Autodesk Inventor part; units mm, degrees
ref_plane "YZ Plane" through (0, 0, 0) normal (1, 0, 0) x (0, 1, 0)
ref_plane "XZ Plane" through (0, 0, 0) normal (0, 1, 0) x (-1, 0, 0)
ref_plane "XY Plane" through (0, 0, 0) normal (0, 0, 1) x (1, 0, 0)
sketch "Esboço1" plane through (0, 0, 0) normal (0, 0, 1) x (1, 0, 0)
  circle A0 centre (0, 0) radius 25
  dimension "d0" = 50
extrude "Extrusão1" add sketch "Esboço1" along normal blind 20
fillet "Arredondamento1" radius 2 1 edges at (-25, 0, 20)
sketch "Esboço2" plane through (0, 0, 20) normal (0, 0, 1) x (1, 0, 0)
  circle A0 centre (0, 0) radius 2.5
  circle A1 centre (0, 18) radius 2.5
  dimension "d4" = 5
  dimension "d5" = 5
  dimension "d6" = 18
extrude "Extrusão2" cut sketch "Esboço2" against normal blind 15
chamfer "Chanfro1" distance 0.6 angle 45 2 edges at (-2.5, 0, 20) (-2.5, 18, 20)
pattern_circular "Padrão circular1" count 6 over 360 about axis through (0, 0, 0) along (0, 0, 1) of "Extrusão2", "Chanfro1"
sketch "Esboço3" plane through (0, 0, 0) normal (0, 0, -1) x (-1, 0, 0)
  arc A0 (3, 30) -> (-3, 30) centre (0, 30) ccw
  circle A1 centre (0, 30) radius 1.5
  line L0 (3, 30) -> (3, 24.3841)
  line L1 (-3, 30) -> (-3, 24.3841)
  line L2 (-3, 24.3841) -> (3, 24.3841)
  point P0 (0, 0)
  dimension "d15" = 6
  dimension "d16" = 3
  dimension "d17" = 30
extrude "Extrusão3" add sketch "Esboço3" against normal blind 5
mirror "Espelhamento1" about plane through (0, 0, 0) normal (0, 1, 0) of "Extrusão3"
sketch "Esboço4" plane through (0, 0, 20) normal (0, 0, 1) x (1, 0, 0)
  circle A0 centre (0, 0) radius 3.1
sketch "Esboço5" plane through (0, 0, 20) normal (0, 0, 1) x (1, 0, 0)
  circle A0 centre (0, 18) radius 3.1
sketch "Esboço6" plane through (0, 0, 20) normal (0, 0, 1) x (1, 0, 0)
  circle A0 centre (15.5885, 9) radius 3.1
sketch "Esboço7" plane through (0, 0, 20) normal (0, 0, 1) x (1, 0, 0)
  circle A0 centre (15.5885, -9) radius 3.1
sketch "Esboço8" plane through (0, 0, 20) normal (0, 0, 1) x (1, 0, 0)
  circle A0 centre (0, -18) radius 3.1
sketch "Esboço9" plane through (0, 0, 20) normal (0, 0, 1) x (1, 0, 0)
  circle A0 centre (-15.5885, -9) radius 3.1
sketch "Esboço10" plane through (0, 0, 20) normal (0, 0, 1) x (1, 0, 0)
  circle A0 centre (-15.5885, 9) radius 3.1
properties part number "Conector2"
CAD build for the part. Positions are in the model's coordinates, mm. A direction names the side the tool comes from. Round coordinates to 2 decimals unless told otherwise and drop trailing zeros. Order: outer loops, then holes, each group sorted by start corner. A loop starts at its lowest first (then second) coordinate and runs counter-clockwise, first axis right, second up.
Q1. Wall check: L1, parallel to Y at x = 0, z = 3.2; L2, parallel to Y at x = 0, z = 14.75; L3, parallel to Y at x = 15.5, z = 18.25. Give the ranges that are in metal, low to high.
Q2. Slice it at C-C (y = 0). Write the cut outline in (x, z).
Q3. Two-plate mould, pull along X, no slides. Class faces 1 (the flat face through (0, -5, 20)), 2 (the flat face through (-3, -27, 2)), 3 (the cylindrical face through (-13.09, 8.89, 12.3)): pulls with the +X half, pulls with the -X half, needs draft (parallel to the pull), parting line crosses it, or undercut.
Q4. Slice it at B-B (z = 14.5). Write the cut outline in (x, y).
Q5. Drop flat-ended pins along their axis: pin 1 (5 mm diameter, centred on x = -1, y = 29.5, fed in from +Z); pin 2 (8 mm diameter, centred on y = 18, z = 9, fed in from -X); pin 3 (2 mm diameter, centred on x = -17, z = 4, fed in from +Y). Give the stop position or say it passes through.
Q6. Which spindle directions (+Z, -Z, +X, -X, +Y, -Y) get a long thin tool onto all of the face, cutting with end or side? Do faces 4 (the flat face through (0, 0, 0)), 5 (the cylindrical face through (-17.43, -7.31, 12.3)). Say none if no direction does.
Q7. Slice it at A-A (z = 2.25). Write the cut outline in (x, y).
Results below:
1. L1: y = -33 to -31.5, -28.5 to 28.5, 31.5 to 33
1. L2: y = -25 to -20.5, -15.5 to -2.5, 2.5 to 15.5, 20.5 to 25
1. L3: y = -19.6 to -11.5, -6.5 to 6.5, 11.5 to 19.6
2. outline: (-25, 0) - (25, 0) - (25, 18) arc R2 ccw to (23, 20) - (3.1, 20) - (2.5, 19.4) - (2.5, 5) - (-2.5, 5) - (-2.5, 19.4) - (-3.1, 20) - (-23, 20) arc R2 ccw to (-25, 18) - close
3. face 1: needs draft
3. face 2: pulls with the -X half
3. face 3: undercut
4. outline: circle Ø50 at (0, 0); hole circle Ø5 at (-15.59, -9); hole circle Ø5 at (-15.59, 9); hole circle Ø5 at (0, -18); hole circle Ø5 at (0, 0); hole circle Ø5 at (0, 18); hole circle Ø5 at (15.59, -9); hole circle Ø5 at (15.59, 9)
5. pin 1: stops at z = 5
5. pin 2: stops at x = -20.71
5. pin 3: stops at y = 19.21
6. face 4: -Z, +X, -X, +Y, -Y
6. face 5: +Z
7. outline: (-3, -30) arc R3 ccw to (3, -30) - (3, -24.82) arc R25 ccw to (3, 24.82) - (3, 30) arc R3 ccw to (-3, 30) - (-3, 24.82) arc R25 ccw to (-3, -24.82) - close; hole circle Ø3 at (0, -30); hole circle Ø3 at (0, 30)
